from build123d import *

# Parameters (mm, degrees)
SKETCH5_R          = 25
CUT_EXTRUDE2_DEPTH = 100


with BuildPart() as part:
    # Sketch4 → Revolve2 (revolve)
    with BuildSketch(Plane.XY, mode=Mode.PRIVATE) as revolve2_sk:
        Polygon((0, -1654.544205968), (300, -1654.544205968), (300, -1554.544205968), (150, -1554.544205968), (150, 345.455794032), (50, 345.455794032), (50, 245.455794032), (0, 245.455794032), align=None)
    revolve(revolve2_sk.sketch.rotate(Axis((0, -1654.544205968, 0), (0, 1, 0)), 90), axis=Axis((0, -1654.544205968, 0), (0, 1, 0)))

    # Sketch5 → Cut-Extrude2 (cut)
    with BuildSketch(Plane(origin=(0, -1554.544205968, 0), x_dir=(1, 0, 0), z_dir=(0, 1, 0))):
        with Locations(Location((0, 255.365455535, 0), (0, 0, 270))):
            Circle(SKETCH5_R)
        with Locations(Location((255.365455535, 0, 0), (0, 0, 270))):
            Circle(SKETCH5_R)
        with Locations(Location((0, -255.365455535, 0), (0, 0, 270))):
            Circle(SKETCH5_R)
        with Locations(Location((-255.365455535, 0, 0), (0, 0, 270))):
            Circle(SKETCH5_R)
    extrude(amount=-CUT_EXTRUDE2_DEPTH, mode=Mode.SUBTRACT)


solid = part.part
Build history of the part. All positions in model axes, mm. A direction names the side the tool comes from. Give positions to 0.01 mm unless a question says otherwise; leave off trailing zeros. Loops run counter-clockwise (first coordinate to the right, second up) from the corner with the lowest first, then second, coordinate; pieces in that order, holes last. Notation, with made-up numbers: (-33.5, 76.5) - (12.5, 76.5) arc R34 cw to (12.5, 106.5) - close; hole circle Ø1 at (-23, -32.75). An arc over 180 degrees is marked (long way). Write item = value, one per line. Start each with the question number.
1) Band-saw the part on C-C on z = -256.5. Give the cut face in (x, y).
2) Pull direction X, two halves, no side cores. Call faces 3 (the flat face through (-4, -1654.544, -4)), 4 (the cylindrical face through (266.152, -1603.844, -138.432)), 5 (the flat face through (-1, 245.456, 1)): +X half, -X half, draft (parallel to the pull), parting line (faces both ways), or undercut.
3) Drop flat-ended pins along their axis: pin 1 Ø12 at (x, z) = (137.5, -78.5) entering from +Y; pin 2 Ø3 at (x, y) = (-32.5, -1431) entering from +Z; pin 3 Ø3 at (y, z) = (-690.5, 54.5) entering from +X. Give the stop position or say it passes through.
4) Band-saw the part on A-A on z = 0. Give the cut face in (x, y), plus the area to 3 significant figures.
5) Band-saw the part on B-B on x = 0. Give the cut face in (y, z), plus the area to 3 significant figures.
6) Probe probe 1 along X at (y, z) = (-1599, 0); probe 2 along X at (y, z) = (282, 0); probe 3 along Y at (x, z) = (88, 162). List the from-to ranges inside material, lowest first. Write a range as from..to.
7) Tool access for faces 1 (the cylindrical face through (-15.02, 294.76, -47.69)), 2 (the flat face through (65, 345.456, 2)): list every direction of +Z, -Z, +X, -X, +Y, -Y with a clear straight run to the whole face (end or side of a thin tool).
8) Band-saw the part on D-D on y = -846. Give the cut face in (x, z).
Final values:
q1.outline = (-155.59, -1654.54) - (-24.97, -1654.54) - (-24.97, -1554.54) - (-155.59, -1554.54) - close; (24.97, -1654.54) - (155.59, -1654.54) - (155.59, -1554.54) - (24.97, -1554.54) - close
q2.face_3 = draft
q2.face_4 = parting line
q2.face_5 = undercut
q3.pin_1 = -1554.54
q3.pin_2 = 146.76
q3.pin_3 = 140.32
q4.outline = (-300, -1654.54) - (-280.37, -1654.54) - (-280.37, -1554.54) - (-300, -1554.54) - close; (-230.37, -1654.54) - (230.37, -1654.54) - (230.37, -1554.54) - (150, -1554.54) - (150, 345.46) - (50, 345.46) - (50, 245.46) - (-50, 245.46) - (-50, 345.46) - (-150, 345.46) - (-150, -1554.54) - (-230.37, -1554.54) - close; (280.37, -1654.54) - (300, -1654.54) - (300, -1554.54) - (280.37, -1554.54) - close
q4.area = 610,000 mm²
q5.outline = (-1654.54, -300) - (-1554.54, -300) - (-1554.54, -280.37) - (-1654.54, -280.37) - close; (-1654.54, -230.37) - (-1554.54, -230.37) - (-1554.54, -150) - (345.46, -150) - (345.46, -50) - (245.46, -50) - (245.46, 50) - (345.46, 50) - (345.46, 150) - (-1554.54, 150) - (-1554.54, 230.37) - (-1654.54, 230.37) - close; (-1654.54, 280.37) - (-1554.54, 280.37) - (-1554.54, 300) - (-1654.54, 300) - close
q5.area = 610,000 mm²
q6.probe_1 = -300..-280.37, -230.37..230.37, 280.37..300
q6.probe_2 = -150..-50, 50..150
q6.probe_3 = -1654.54..-1554.54
q7.face_1 = +Y
q7.face_2 = +Z, -Z, +X, -X, +Y
q8.outline = circle Ø300 at (0, 0)
